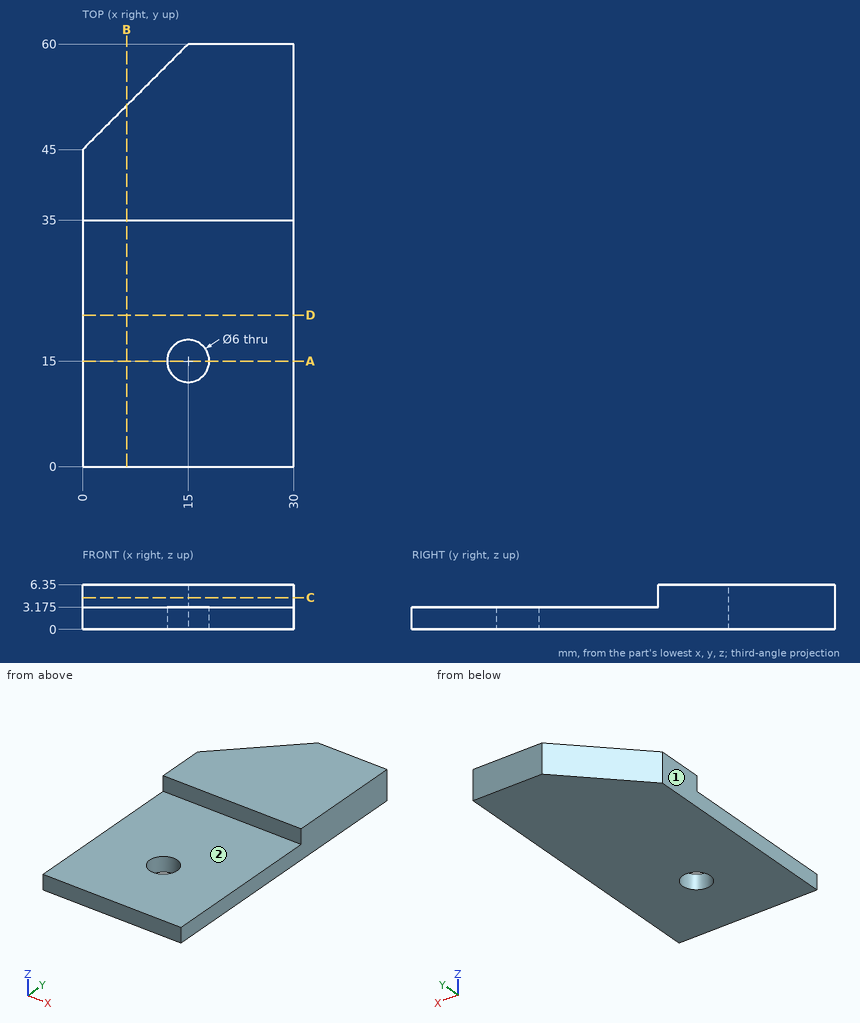
Could you check a few things on this drawing? It's one solid part, dimensions in mm from its lowest x, y, z. A direction names the side the tool comes from. Give positions to 0.01 mm unless a question says otherwise; leave off trailing zeros. Loops run counter-clockwise (first coordinate to the right, second up) from the corner with the lowest first, then second, coordinate; pieces in that order, holes last. Notation, with made-up numbers: (54, 21) -> (106, 21) arc R20 ccw to (106, 40) -> close; hole circle Ø9 at (-31.5, 20). An arc over 180 degrees is marked (long way). Use one line per item in the form item = value. Start each with the question number.
1) Imagine slicing it at C-C (z = 4.5). Please give me the cut outline in (x, y).
2) Which directions (+Z, -Z, +X, -X, +Y, -Y) give clear straight access to the entire face, cutting with the end or side of a thin tool? Please do the marked faces 1 and 2.
3) Imagine slicing it at B-B (x = 6.25). Please give me the cut outline in (y, z) (3 decimals), then the cut area to 3 significant figures.
4) Please list where these lines run through material, in increasing order: line 1 along Z through (x, y) = (12, 24) (3 decimals); line 2 along Y through (x, z) = (28.75, 5.5); line 3 along X through (y, z) = (53, 2.25).
5) Imagine slicing it at A-A (y = 15). Please give me the cut outline in (x, z) (3 decimals).
6) Imagine slicing it at D-D (y = 21.5). Please give me the cut outline in (x, z) (3 decimals).
7) For P1, Ø5, axis at x = 14, y = 10.5, coming from the +Z side (3 decimals); P2, Ø2, axis at x = 13, z = 1.5, coming from the +Y side; P3, Ø3.5, axis at x = 8, z = 5.5, coming from the -Y side, each with a flat end and sliding along its axis, tell me the tip position at first contact or that it passes through.
Check values:
q1.outline = (0, 35) -> (30, 35) -> (30, 60) -> (15, 60) -> (0, 45) -> close
q2.face_1 = +Z, -Z, -X, +Y, -Y
q2.face_2 = +Z, +X, -X, -Y
q3.outline = (0, 0) -> (51.25, 0) -> (51.25, 6.35) -> (35, 6.35) -> (35, 3.175) -> (0, 3.175) -> close
q3.area = 214 mm^2
q4.line_1 = 0 to 3.175
q4.line_2 = 35 to 60
q4.line_3 = 8 to 30
q5.outline = (0, 0) -> (12, 0) -> (12, 3.175) -> (0, 3.175) -> close; (18, 0) -> (30, 0) -> (30, 3.175) -> (18, 3.175) -> close
q6.outline = (0, 0) -> (30, 0) -> (30, 3.175) -> (0, 3.175) -> close
q7.P1 = 3.175
q7.P2 = 59
q7.P3 = 35
